from build123d import *

# Parameters (mm, degrees)
SKETCH1_R           = 17.5
BOSS_EXTRUDE1_DEPTH = 5
SKETCH2_R           = 14
BOSS_EXTRUDE2_DEPTH = 155
SKETCH3_R           = 10
CUT_EXTRUDE2_DEPTH  = 150
SKETCH4_W           = 30
SKETCH4_H           = 30
BOSS_EXTRUDE3_DEPTH = 15
SKETCH5_W           = 30
SKETCH5_H           = 16
CUT_EXTRUDE3_DEPTH  = 15
SKETCH6_R           = 4
CUT_EXTRUDE4_DEPTH  = 30


with BuildPart() as part:
    # Sketch1 → Boss-Extrude1 (new body)
    with BuildSketch(Plane.XY):
        Circle(SKETCH1_R)
    extrude(amount=BOSS_EXTRUDE1_DEPTH)

    # Sketch2 → Boss-Extrude2 (add)
    with BuildSketch(Plane.XY):
        Circle(SKETCH2_R)
    extrude(amount=BOSS_EXTRUDE2_DEPTH)

    # Sketch3 → Cut-Extrude2 (cut)
    with BuildSketch(Plane.XY.offset(155)):
        Circle(SKETCH3_R)
    extrude(amount=-CUT_EXTRUDE2_DEPTH, mode=Mode.SUBTRACT)

    # Sketch4 → Boss-Extrude3 (add)
    with BuildSketch(Plane.XY.offset(155)):
        Rectangle(SKETCH4_W, SKETCH4_H)
    extrude(amount=BOSS_EXTRUDE3_DEPTH)

    # Sketch5 → Cut-Extrude3 (cut)
    with BuildSketch(Plane.XY.offset(170)):
        Rectangle(SKETCH5_W, SKETCH5_H)
    extrude(amount=-CUT_EXTRUDE3_DEPTH, mode=Mode.SUBTRACT)

    # Sketch6 → Cut-Extrude4 (cut)
    with BuildSketch(Plane(origin=(0, 11.5, 0), x_dir=(1, 0, 0), z_dir=(0, 1, 0))):
        with Locations(Location((0, -162.5, 0), (0, 0, 270))):
            Circle(SKETCH6_R)
    extrude(amount=-CUT_EXTRUDE4_DEPTH, mode=Mode.SUBTRACT)


solid = part.part
Verification items for the finished model (mm, model axes). A direction names the side the tool comes from. Coordinates: 2 decimals unless noted, no trailing zeros. Write each loop counter-clockwise with the first axis right and the second up, starting at its lowest first coordinate (ties: lowest second). Pieces come first, ordered by that corner, then holes. Notation, with made-up numbers: (71, -20) -> (124, -20) arc R10 ccw to (124, -12) -> close; hole circle Ø6 at (64, 65.25). An arc over 180 degrees is marked (long way). One line per item, written item: value. Start each with the question number.
Q1. Cross-section at D-D on z = 83. Enter the section's corners in (x, y).
Q2. Mould release check, pull along Z, two halves, no side actions. Record for faces 6 (the flat face through (-15, -12, 162)), 7 (the flat face through (0, 0, 0)), 8 (the flat face through (-0.2, -14.6, 155)): pulls with the +Z half, pulls with the -Z half, needs draft (parallel to the pull), parting line crosses it, or undercut.
Q3. Cross-section at C-C on y = 0. Enter the section's corners in (x, z).
Q4. Thickness scan on L1, parallel to Y at x = 0, z = 119; L2, parallel to Z at x = 8.5, y = -13; L3, parallel to X at y = -9.5, z = 162.5. Record the ranges inside material, lowest first. Write a range as from..to.
Q5. Cross-section at A-A on z = 162.5. Enter the section's corners in (x, y), and give its area (3 significant figures).
Q6. Cross-section at B-B on x = 0. Enter the section's corners in (y, z).
Q7. Access from +Z, -Z, +X, -X, +Y, -Y to the whole of each face (thin tool, end or side, straight path). Record for faces 1 (the flat face through (-4, -8, 166)), 2 (the flat face through (-4, -15, 159)), 3 (the flat face through (0, 15, 162)), 4 (the flat face through (0, 11.5, 162)), 5 (the flat face through (0, 0, 5)).
Q8. Go/stop test with flat-tipped pins: P1, Ø13, axis at x = 0, z = 162.5, coming from the +Y side; P2, Ø10, axis at y = 2.5, z = 77.5, coming from the -X side; P3, Ø10, axis at y = -7, z = 45, coming from the -X side. Record where each tip stops, or that it passes through.
Checked values:
1. outline: circle Ø28 at (0, 0); hole circle Ø20 at (0, 0)
2. face 6: needs draft
2. face 7: pulls with the -Z half
2. face 8: undercut
3. outline: (-17.5, 0) -> (17.5, 0) -> (17.5, 5) -> (14, 5) -> (14, 155) -> (10, 155) -> (10, 5) -> (-10, 5) -> (-10, 155) -> (-14, 155) -> (-14, 5) -> (-17.5, 5) -> close
4. L1: y = -14..-10, 10..14
4. L2: z = 0..5, 155..170
4. L3: x = -15..-4, 4..15
5. outline: (-15, -15) -> (-4, -15) -> (-4, -8) -> (-15, -8) -> close; (-15, 8) -> (-4, 8) -> (-4, 11.5) -> (4, 11.5) -> (4, 8) -> (15, 8) -> (15, 15) -> (-15, 15) -> close; (4, -15) -> (15, -15) -> (15, -8) -> (4, -8) -> close
5. area: 336 mm²
6. outline: (-17.5, 0) -> (17.5, 0) -> (17.5, 5) -> (14, 5) -> (14, 155) -> (15, 155) -> (15, 170) -> (8, 170) -> (8, 166.5) -> (11.5, 166.5) -> (11.5, 158.5) -> (8, 158.5) -> (8, 155) -> (10, 155) -> (10, 5) -> (-10, 5) -> (-10, 155) -> (-8, 155) -> (-8, 158.5) -> (-15, 158.5) -> (-15, 155) -> (-14, 155) -> (-14, 5) -> (-17.5, 5) -> close; (-15, 166.5) -> (-8, 166.5) -> (-8, 170) -> (-15, 170) -> close
7. face 1: +Z, +X, -X
7. face 2: +Z, +X, -X, -Y
7. face 3: +Z, +X, -X, +Y
7. face 4: -Y
7. face 5: none
8. P1: stops at y = 15
8. P2: stops at x = -14
8. P3: stops at x = -13.86
